Part model, mm, in its own coordinate system. Give positions to 0.01 mm unless a question says otherwise; leave off trailing zeros. Order: outer loops, then holes, each group sorted by start corner. A loop starts at its lowest first (then second) coordinate and runs counter-clockwise, first axis right, second up. Notation, with made-up numbers: M 30,21.5 L 40,21.5 A14 ccw 40,32.5 Z; hole C 57,-4 d1. An arc over 180 degrees is marked long. One line per question, with ' | ' between items.
Autodesk Inventor part; units mm, degrees
ref_plane "YZ Plane" through (0, 0, 0) normal (1, 0, 0) x (0, 1, 0)
ref_plane "XZ Plane" through (0, 0, 0) normal (0, 1, 0) x (-1, 0, 0)
ref_plane "XY Plane" through (0, 0, 0) normal (0, 0, 1) x (1, 0, 0)
sketch "Sketch1" plane through (0, 0, 0) normal (0, 1, 0) x (-1, 0, 0)
  line L0 (-12.5, 26) -> (12.5, 26)
  line L1 (12.5, 26) -> (12.5, 19.2)
  line L2 (8.5, -26) -> (-8.5, -26)
  circle A0 centre (0, 19.6) radius 1.65
  line L3 (0, 26) -> (10.85, 26)
  arc A1 (10.85, 18.2) -> (10.85, 14.8) centre (10.85, 16.5) ccw
  line L4 (10.85, 18.2) -> (11.5, 18.2)
  line L5 (10.85, 14.8) -> (11.5, 14.8)
  arc A2 (11.5, 18.2) -> (12.5, 19.2) centre (11.5, 19.2) ccw
  arc A3 (12.5, 13.8) -> (11.5, 14.8) centre (11.5, 13.8) ccw
  arc A4 (10.85, 11.85) -> (10.85, 8.45) centre (10.85, 10.15) ccw
  line L6 (10.85, 11.85) -> (11.5, 11.85)
  line L7 (10.85, 8.45) -> (11.5, 8.45)
  arc A5 (11.5, 11.85) -> (12.5, 12.85) centre (11.5, 12.85) ccw
  arc A6 (12.5, 7.45) -> (11.5, 8.45) centre (11.5, 7.45) ccw
  arc A7 (10.85, 5.5) -> (10.85, 2.1) centre (10.85, 3.8) ccw
  line L8 (10.85, 5.5) -> (11.5, 5.5)
  line L9 (10.85, 2.1) -> (11.5, 2.1)
  arc A8 (11.5, 5.5) -> (12.5, 6.5) centre (11.5, 6.5) ccw
  arc A9 (12.5, 1.1) -> (11.5, 2.1) centre (11.5, 1.1) ccw
  arc A10 (10.85, -0.85) -> (10.85, -4.25) centre (10.85, -2.55) ccw
  line L10 (10.85, -0.85) -> (11.5, -0.85)
  line L11 (10.85, -4.25) -> (11.5, -4.25)
  arc A11 (11.5, -0.85) -> (12.5, 0.15) centre (11.5, 0.15) ccw
  arc A12 (12.5, -5.25) -> (11.5, -4.25) centre (11.5, -5.25) ccw
  arc A13 (10.85, -7.2) -> (10.85, -10.6) centre (10.85, -8.9) ccw
  line L12 (10.85, -7.2) -> (11.5, -7.2)
  line L13 (10.85, -10.6) -> (11.5, -10.6)
  arc A14 (11.5, -7.2) -> (12.5, -6.2) centre (11.5, -6.2) ccw
  arc A15 (12.5, -11.6) -> (11.5, -10.6) centre (11.5, -11.6) ccw
  arc A16 (10.85, -13.55) -> (10.85, -16.95) centre (10.85, -15.25) ccw
  line L14 (10.85, -13.55) -> (11.5, -13.55)
  line L15 (10.85, -16.95) -> (11.5, -16.95)
  arc A17 (11.5, -13.55) -> (12.5, -12.55) centre (11.5, -12.55) ccw
  arc A18 (12.5, -17.95) -> (11.5, -16.95) centre (11.5, -17.95) ccw
  line L16 (12.5, 13.8) -> (12.5, 12.85)
  line L17 (12.5, 7.45) -> (12.5, 6.5)
  line L18 (12.5, 1.1) -> (12.5, 0.15)
  line L19 (12.5, -5.25) -> (12.5, -6.2)
  line L20 (12.5, -11.6) -> (12.5, -12.55)
  line L21 (12.5, -17.95) -> (12.5, -22)
  line L22 (-12.5, 26) -> (-12.5, 19.2)
  arc A19 (-10.85, 14.8) -> (-10.85, 18.2) centre (-10.85, 16.5) ccw
  line L23 (-10.85, 18.2) -> (-11.5, 18.2)
  line L24 (-10.85, 14.8) -> (-11.5, 14.8)
  arc A20 (-12.5, 19.2) -> (-11.5, 18.2) centre (-11.5, 19.2) ccw
  arc A21 (-11.5, 14.8) -> (-12.5, 13.8) centre (-11.5, 13.8) ccw
  arc A22 (-11.5, 8.45) -> (-12.5, 7.45) centre (-11.5, 7.45) ccw
  line L25 (-10.85, 8.45) -> (-11.5, 8.45)
  line L26 (-10.85, 11.85) -> (-11.5, 11.85)
  arc A23 (-12.5, 12.85) -> (-11.5, 11.85) centre (-11.5, 12.85) ccw
  arc A24 (-10.85, 8.45) -> (-10.85, 11.85) centre (-10.85, 10.15) ccw
  arc A25 (-11.5, 2.1) -> (-12.5, 1.1) centre (-11.5, 1.1) ccw
  line L27 (-10.85, 2.1) -> (-11.5, 2.1)
  line L28 (-10.85, 5.5) -> (-11.5, 5.5)
  arc A26 (-12.5, 6.5) -> (-11.5, 5.5) centre (-11.5, 6.5) ccw
  arc A27 (-10.85, 2.1) -> (-10.85, 5.5) centre (-10.85, 3.8) ccw
  arc A28 (-11.5, -4.25) -> (-12.5, -5.25) centre (-11.5, -5.25) ccw
  line L29 (-10.85, -4.25) -> (-11.5, -4.25)
  line L30 (-10.85, -0.85) -> (-11.5, -0.85)
  arc A29 (-12.5, 0.15) -> (-11.5, -0.85) centre (-11.5, 0.15) ccw
  arc A30 (-10.85, -4.25) -> (-10.85, -0.85) centre (-10.85, -2.55) ccw
  arc A31 (-11.5, -10.6) -> (-12.5, -11.6) centre (-11.5, -11.6) ccw
  line L31 (-10.85, -10.6) -> (-11.5, -10.6)
  line L32 (-10.85, -7.2) -> (-11.5, -7.2)
  arc A32 (-12.5, -6.2) -> (-11.5, -7.2) centre (-11.5, -6.2) ccw
  arc A33 (-10.85, -10.6) -> (-10.85, -7.2) centre (-10.85, -8.9) ccw
  arc A34 (-11.5, -16.95) -> (-12.5, -17.95) centre (-11.5, -17.95) ccw
  line L33 (-10.85, -16.95) -> (-11.5, -16.95)
  line L34 (-10.85, -13.55) -> (-11.5, -13.55)
  arc A35 (-12.5, -12.55) -> (-11.5, -13.55) centre (-11.5, -12.55) ccw
  arc A36 (-10.85, -16.95) -> (-10.85, -13.55) centre (-10.85, -15.25) ccw
  line L35 (-12.5, 13.8) -> (-12.5, 12.85)
  line L36 (-12.5, 7.45) -> (-12.5, 6.5)
  line L37 (-12.5, 1.1) -> (-12.5, 0.15)
  line L38 (-12.5, -5.25) -> (-12.5, -6.2)
  line L39 (-12.5, -11.6) -> (-12.5, -12.55)
  line L40 (-12.5, -17.95) -> (-12.5, -22)
  arc A37 (8.5, -26) -> (12.5, -22) centre (8.5, -22) ccw
  arc A38 (-12.5, -22) -> (-8.5, -26) centre (-8.5, -22) ccw
  circle A39 centre (0, 13.25) radius 1.65
  circle A40 centre (0, 6.9) radius 1.65
  circle A41 centre (0, 0.55) radius 1.65
  circle A42 centre (0, -5.8) radius 1.65
  circle A43 centre (0, -12.15) radius 1.65
  circle A44 centre (0, -18.5) radius 1.65
  point P0 (-12.5, -26)
  point P1 (12.5, -26)
  point P2 (12.5, 14.8)
  point P3 (12.5, 8.45)
  point P4 (12.5, 2.1)
  point P5 (12.5, -4.25)
  point P6 (12.5, -10.6)
  point P7 (12.5, -16.95)
  point P8 (-12.5, 14.8)
  point P9 (-12.5, 8.45)
  point P10 (-12.5, 2.1)
  point P11 (-12.5, -4.25)
  point P12 (-12.5, -10.6)
  point P13 (-12.5, -16.95)
  dimension "d0" = 52
  dimension "d1" = 25
  dimension "d3" = 3.3
  dimension "d16" = 10.85
  dimension "d18" = 1.7
  dimension "d19" = 1
  dimension "d20" = 1
  dimension "d22" = 1.7
  dimension "d23" = 1
  dimension "d24" = 1
  dimension "d26" = 1.7
  dimension "d27" = 1
  dimension "d28" = 1
  dimension "d30" = 1.7
  dimension "d31" = 1
  dimension "d32" = 1
  dimension "d34" = 1.7
  dimension "d35" = 1
  dimension "d36" = 1
  dimension "d38" = 1.7
  dimension "d39" = 1
  dimension "d40" = 1
  dimension "d42" = 4
  dimension "d44" = 3.3
  dimension "d46" = 3.3
  dimension "d48" = 3.3
  dimension "d50" = 3.3
  dimension "d52" = 3.3
  dimension "d54" = 3.3
extrude "Extrusion1" add sketch "Sketch1" along normal blind 2
fillet "Fillet2" radius 2 2 edges at (12.5, 1, 26) (-12.5, 1, 26)
properties part number "Motor Mount Bracket" material "Acrylic"
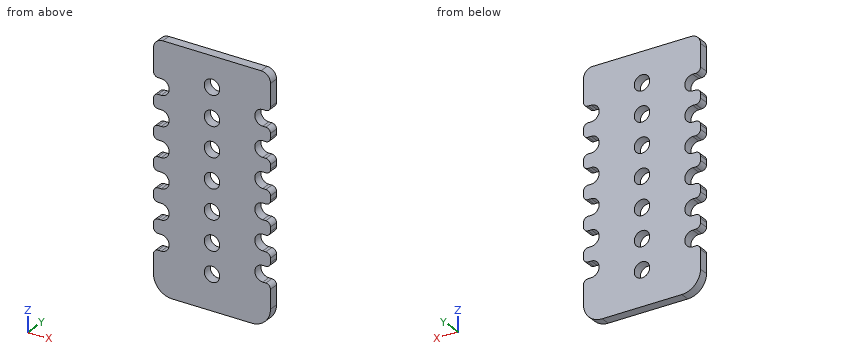
1. Slice it at A-A on x = 0. Give the number of separate pieces and of enclosed holes in the cut face, then the cut area to 3 significant figures.
Worked out:
separate pieces: 8 | enclosed holes: 0 | area: 57.8 mm2
2. Slice it at C-C on x = 9.75. Give the cut face in (y, z).
Worked out:
outline: M 0,-25.8 L 2,-25.8 L 2,-16.55 L 0,-16.55 Z; M 0,-13.95 L 2,-13.95 L 2,-10.2 L 0,-10.2 Z; M 0,-7.6 L 2,-7.6 L 2,-3.85 L 0,-3.85 Z; M 0,-1.25 L 2,-1.25 L 2,2.5 L 0,2.5 Z; M 0,5.1 L 2,5.1 L 2,8.85 L 0,8.85 Z; M 0,11.45 L 2,11.45 L 2,15.2 L 0,15.2 Z; M 0,17.8 L 2,17.8 L 2,26 L 0,26 Z
3. Slice it at B-B on z = -18.5. Give the cut face in (x, y).
Worked out:
outline: M -12.5,0 L -1.65,0 L -1.65,2 L -12.5,2 Z; M 1.65,0 L 12.5,0 L 12.5,2 L 1.65,2 Z
4. Probe L1, parallel to X at y = 0.9, z = -6; L2, parallel to X at y = 1.35, z = 4; L3, parallel to X at y = 0.9, z = 20.5. List the from-to ranges inside material, lowest first. Write a range as from..to.
Worked out:
L1: x = -12.5..-1.64, 1.64..12.5 | L2: x = -9.16..9.16 | L3: x = -12.5..-1.38, 1.38..12.5
5. Drop flat-ended pins along their axis: pin 1 (0.5 mm diameter, centred on x = -11.5, y = 1, fed in from +Z); pin 2 (0.7 mm diameter, centred on x = 11, y = 1, fed in from -Z); pin 3 (0.7 mm diameter, centred on x = 11, y = 1, fed in from +Z). Give the stop position or say it passes through.
Worked out:
pin 1: stops at z = 25.85 | pin 2: stops at z = -25.37 | pin 3: stops at z = 25.99
